Answer from the drawing. Dimensions are ordinates in mm from the lowest x, y and z of the part. Round coordinates to 2 decimals unless told otherwise and drop trailing zeros. Loops run counter-clockwise (first coordinate to the right, second up) from the corner with the lowest first, then second, coordinate; pieces in that order, holes last.
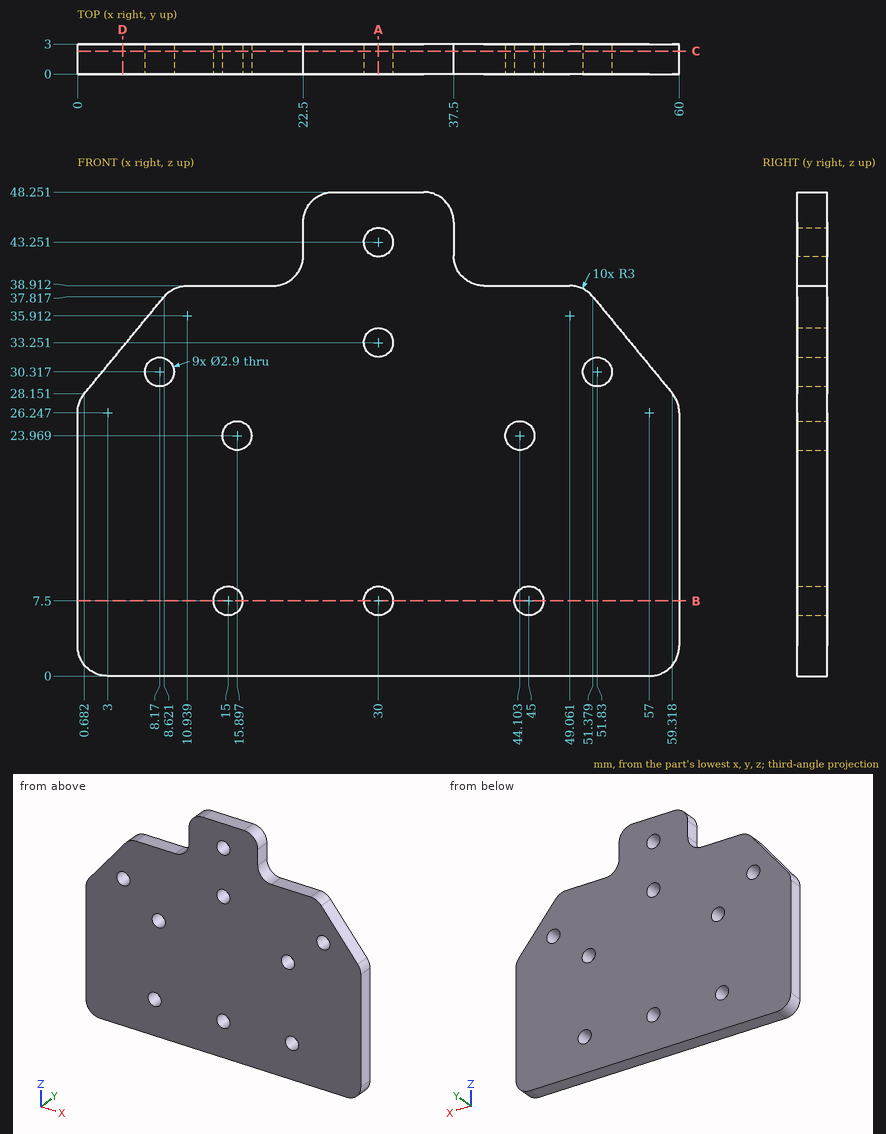
1. Find section C-C (y = 2.3). Give the number of separate pieces and of enclosed holes in the cut face, then the cut area to 3 significant figures.
Answer key:
separate pieces: 1
enclosed holes: 9
area: 2,300 mm2
2. Find section A-A (x = 30). Write down the section's boundary in (y, z).
Answer key:
outline: (0, 0) - (3, 0) - (3, 6.05) - (0, 6.05) - close; (0, 8.95) - (3, 8.95) - (3, 31.8) - (0, 31.8) - close; (0, 34.7) - (3, 34.7) - (3, 41.8) - (0, 41.8) - close; (0, 44.7) - (3, 44.7) - (3, 48.25) - (0, 48.25) - close
3. Given pin 1 (0.9 mm diameter, centred on y = 1, z = 43, fed in from +X); pin 2 (1.5 mm diameter, centred on y = 1.5, z = 43, fed in from -X); pin 3 (1.7 mm diameter, centred on x = 30, z = 7.5, fed in from -Y); pin 4 (1.5 mm diameter, centred on x = 13.5, y = 1, fed in from +Z), each flat-ended and moving along its own axis, determine where each tip first touches the part or whether it passes through.
Answer key:
pin 1: stops at x = 37.5
pin 2: stops at x = 22.5
pin 3: passes through
pin 4: stops at z = 38.91
4. Find section D-D (x = 4.5). Write down the section's boundary in (y, z).
Answer key:
outline: (0, 0) - (3, 0) - (3, 32.8) - (0, 32.8) - close
5. Consider probe 1 along X at (y, z) = (1.3, 7.5); probe 2 along X at (y, z) = (2.85, 23.5) (1 decimal); probe 3 along Z at (x, y) = (45, 1.5). Determine where each line is inside the solid, lowest interval first.
Answer key:
probe 1: x = 0 to 13.55, 16.45 to 28.55, 31.45 to 43.55, 46.45 to 60
probe 2: x = 0 to 14.5, 17.3 to 42.7, 45.5 to 60
probe 3: z = 0 to 6.05, 8.95 to 22.83, 25.11 to 38.91
6. Find section B-B (z = 7.5). Write down the section's boundary in (x, y), then the cut area to 3 significant figures.
Answer key:
outline: (0, 0) - (13.55, 0) - (13.55, 3) - (0, 3) - close; (16.45, 0) - (28.55, 0) - (28.55, 3) - (16.45, 3) - close; (31.45, 0) - (43.55, 0) - (43.55, 3) - (31.45, 3) - close; (46.45, 0) - (60, 0) - (60, 3) - (46.45, 3) - close
area: 154 mm2
